For this review, take the finished solid that the model builds, in its own axes (mm). Face numbers are marked on the shaded views. Round coordinates to 2 decimals unless told otherwise and drop trailing zeros. Loops run counter-clockwise (first coordinate to the right, second up) from the corner with the lowest first, then second, coordinate; pieces in that order, holes last.
1. Consider section D-D on y = 49.5. State the section outline as (x, z) points, then the cut area to 3 significant figures.
2. Consider section C-C on z = 10. State the section outline as (x, y) points.
3. Consider section B-B on x = 283. State the section outline as (y, z) points.
4. Clearance check with flat-ended pins moving along their axes: pin 1 Ø8.5 at (x, z) = (213.5, 6.5) entering from -Y; pin 2 Ø6 at (y, z) = (60, 36) entering from -X; pin 3 Ø12 at (y, z) = (58.5, 73.5) entering from +X; pin 4 Ø5 at (x, y) = (247.5, 20.5) entering from +Z. State where each tip first meets the part, or that it passes through.
5. To check wall thickness, follow line 1 along Z through (x, y) = (232, 39); line 2 along X through (y, z) = (60, 21); line 3 along Y through (x, z) = (300, 27.5). State the ranges of each line that lie inside material, in increasing order.
6. Draft analysis for pull direction X (two halves, no side actions). For the marked faces 1, 2 and 3, state which applies: released by +X, released by -X, zero draft, split by the parting line, or undercut.
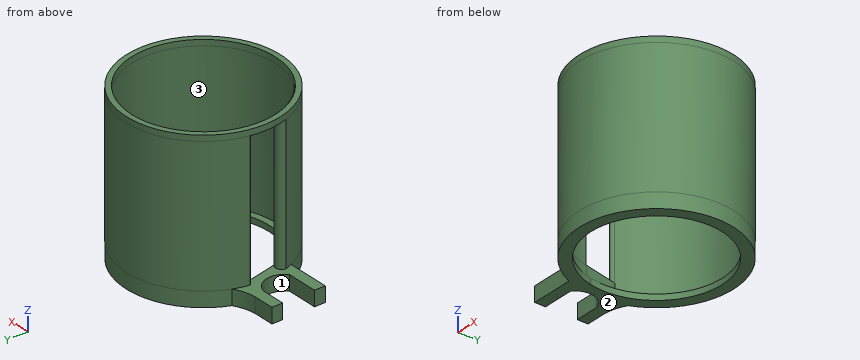
from build123d import *

# Parameters (mm, degrees)
PAD002_DEPTH  = 7.8
PAD_DEPTH     = 70
SKETCH037_R   = 40
SKETCH037_R_2 = 37.263874
PAD003_DEPTH  = 3
SKETCH038_R   = 37.75
SKETCH038_R_2 = 34.1163531471
PAD004_DEPTH  = 3


with BuildPart() as part:
    # Sketch036 → Pad002 (new body)
    with BuildSketch(Plane.XY.offset(4.25)):
        with BuildLine():
            Line((221.1908881172, 52.117988), (210.2803272855, 52.117988))
            Line((210.2803272855, 52.117988), (210.2803272855, 46.517988))
            Line((210.2803272855, 46.517988), (222.4393319888, 46.517988))
            ThreePointArc((226.517548, 30.017988), (229.5828812778, 39.5296252224), (222.4393319888, 46.517988))
            Line((220.1803272855, 30.017988), (226.517548, 30.017988))
            Line((210.2803272855, 30.017988), (220.1803272855, 30.017988))
            Line((210.2803272855, 30.017988), (210.2803272855, 24.417988))
            Line((210.2803272855, 24.417988), (232.4311698855, 24.417988))
            ThreePointArc((232.4311698855, 24.417988), (309.0297689267, 41.1984446323), (231.9255099311, 55.4764817733))
            ThreePointArc((221.1908881172, 52.117988), (226.7588734106, 53.1558272223), (231.9255099311, 55.4764817733))
        make_face()
        with BuildLine():
            ThreePointArc((252.5144646184, 6.8824824424), (302.747151692, 56.9712258563), (232.3426033937, 48.2876409781))
            Line((236.38045916, 30.2532447879), (232.3426033937, 48.2876409781))
            ThreePointArc((236.38045916, 30.2532447879), (242.114784508, 16.9574998176), (252.5144646184, 6.8824824424))
        make_face(mode=Mode.SUBTRACT)
    extrude(amount=PAD002_DEPTH)

    # Sketch (on Face15 of Pad002) → Pad (join)
    with BuildSketch(Plane.XY.offset(12.05)):
        with BuildLine():
            ThreePointArc((252.4808381991, 6.8990050545), (302.7374672811, 56.9910894012), (232.3258342856, 48.2077176229))
            ThreePointArc((229.7781905775, 48.2217645891), (231.0448692794, 46.9192153434), (232.3258342856, 48.2077176229))
            ThreePointArc((230.9504948913, 28.3176101637), (308.9658709648, 42.8991184314), (229.7781905775, 48.2217645891))
            ThreePointArc((236.4314409979, 30.017988), (233.1244202603, 30.9939916247), (230.9504948913, 28.3176101637))
            ThreePointArc((236.4314409979, 30.017988), (242.1720253216, 16.8728447116), (252.4808381991, 6.8990050545))
        make_face()
    extrude(amount=PAD_DEPTH)

    # Sketch037 (on Face21 of Pad) → Pad003 (join)
    with BuildSketch(Plane.XY.offset(82.05)):
        with Locations((269.0350692214, 40.5472952824)):
            Circle(SKETCH037_R)
        with Locations((269.0350692214, 40.5472952824)):
            Circle(SKETCH037_R_2, mode=Mode.SUBTRACT)
    extrude(amount=PAD003_DEPTH)

    # Sketch038 → Pad004 (join)
    with BuildSketch(Plane.XY.offset(4.25)):
        with Locations((269.0350692214, 40.5472952824)):
            Circle(SKETCH038_R)
        with Locations((269.0350692214, 40.5472952824)):
            Circle(SKETCH038_R_2, mode=Mode.SUBTRACT)
    extrude(amount=PAD004_DEPTH)


solid = part.part
Resolved:
1. outline: (210.28, 4.25) - (236.11, 4.25) - (236.11, 7.25) - (232.62, 7.25) - (232.62, 82.05) - (232.86, 82.05) - (232.86, 85.05) - (230.05, 85.05) - (230.05, 12.05) - (210.28, 12.05) - close; (301.96, 4.25) - (308.02, 4.25) - (308.02, 85.05) - (305.21, 85.05) - (305.21, 82.05) - (305.45, 82.05) - (305.45, 7.25) - (301.96, 7.25) - close
1. area: 592 mm2
2. outline: (210.28, 24.42) - (232.43, 24.42) arc R40 ccw (long way) to (231.93, 55.48) arc R23.87 cw to (221.19, 52.12) - (210.28, 52.12) - (210.28, 46.52) - (222.44, 46.52) arc R9.5 cw to (226.52, 30.02) - (210.28, 30.02) - close; hole (232.34, 48.29) - (236.38, 30.25) arc R36.98 ccw to (252.51, 6.88) arc R37.5 ccw (long way) to start
3. outline: (3.06, 4.25) - (9.42, 4.25) - (9.42, 7.25) - (5.74, 7.25) - (5.74, 82.05) - (6, 82.05) - (6, 85.05) - (3.06, 85.05) - close; (71.67, 4.25) - (78.03, 4.25) - (78.03, 85.05) - (75.1, 85.05) - (75.1, 82.05) - (75.35, 82.05) - (75.35, 7.25) - (71.67, 7.25) - close
4. pin 1: stops at y = 24.42
4. pin 2: stops at x = 232.58
4. pin 3: stops at x = 307.21
4. pin 4: passes through
5. line 1: z = 4.25 to 12.05
5. line 2: x = 234.08 to 236.98, 301.1 to 303.99
5. line 3: y = 15.23 to 19.39, 61.7 to 65.87
6. face 1: released by -X
6. face 2: zero draft
6. face 3: undercut
